Here's how the part is built. I have some questions about the finished solid (model axes, mm). A direction names the side the tool comes from. Coordinates: 2 decimals unless noted, no trailing zeros. Use a Markdown table: item, result. Add a question column.
Item 1: If we mould it in two halves opening along Z, with no side actions, what happens to faces 3 (the flat face through (91.03, -157.32, -249.72)), 4 (the cylindrical face through (-12.77, -1.27, 0.28)), 5 (the flat face through (91.03, -157.32, 249.72))? For each: pulls with the +Z half, pulls with the -Z half, needs draft (parallel to the pull), parting line crosses it, or undercut.
Item 2: If I drill on line 1 along Y through (x, z) = (41, 180); line 2 along Y through (x, z) = (28, -139); line 3 along X through (y, z) = (-101.5, -154), over which ranges is the centre line in solid material (lowest first)? Write a range as from..to.
Item 3: Will these pins go through, and if not, where does the flat tip stop? pin 1 Ø11 at (x, z) = (8.5, 7) entering from +Y; pin 2 Ø4 at (x, z) = (-30.5, 4.5) entering from -Y; pin 3 Ø12.5 at (x, y) = (-18.5, 5) entering from +Z.
Item 4: On a 3-axis mill with a long thin cutter (end or side, diameter ignored), from which of +Z, -Z, +X, -X, +Y, -Y can I reach the whole of each face in a straight line? I mean faces 1 (the flat face through (-12, 2, -20.32)), 2 (the cylindrical face through (-6.17, 25.95, -0.37)). Say none if no direction works.
```python
from build123d import *

# Parameters (mm, degrees)
BOSS_EXTRUDE1_DEPTH = 10.16
SKETCH2_OUTSIDE_W   = 88.516
SKETCH2_OUTSIDE_H   = 38.986
CUT_EXTRUDE1_DEPTH  = 41.64
SKETCH3_R           = 12.7


with BuildPart() as part:
    # Sketch1 → Boss-Extrude1 (new body, symmetric)
    with BuildSketch(Plane(origin=(0, 0, 0), x_dir=(1, 0, 0), z_dir=(0, 1, 0))):
        with BuildLine():
            Line((4.607085175, 20.32), (-28.448, 20.32))
            ThreePointArc((-28.448, 20.32), (-32.938128061, 18.460128061), (-34.798, 13.97))
            Line((-34.798, 13.97), (-34.798, -13.97))
            ThreePointArc((-34.798, -13.97), (-32.938128061, -18.460128061), (-28.448, -20.32))
            Line((-28.448, -20.32), (4.607085175, -20.32))
            ThreePointArc((4.607085175, -20.32), (10.031876423, -19.733940435), (15.206332963, -18.002806293))
            Line((15.206332963, -18.002806293), (30.611774336, -10.928879131))
            ThreePointArc((30.611774336, -10.928879131), (33.846603668, -8.117096905), (35.052, -4.004037244))
            Line((35.052, -4.004037244), (35.052, 4.004037244))
            ThreePointArc((35.052, 4.004037244), (33.846603668, 8.117096905), (30.611774336, 10.928879131))
            Line((30.611774336, 10.928879131), (15.206332963, 18.002806293))
            ThreePointArc((15.206332963, 18.002806293), (10.031876423, 19.733940435), (4.607085175, 20.32))
        make_face()
    extrude(amount=BOSS_EXTRUDE1_DEPTH, both=True)

    # Sketch2 outside → Cut-Extrude1 (cut, through all)
    with BuildSketch(Plane.XY.offset(20.32)):
        with Locations((0.127, 0)):
            Rectangle(SKETCH2_OUTSIDE_W, SKETCH2_OUTSIDE_H)
        with BuildLine():
            Line((-34.798, 10.16), (-24.638, 10.16))
            ThreePointArc((-24.638, 10.16), (-12.998257735, 2.54), (-1.35851547, 10.16))
            Line((-1.35851547, 10.16), (35.052, 10.16))
            Line((35.052, 10.16), (35.052, 6.35))
            Line((35.052, 6.35), (0.913895226, 6.35))
            ThreePointArc((0.913895226, 6.35), (-12.998257735, -1.27), (-26.910410695, 6.35))
            Line((-26.910410695, 6.35), (-34.798, 6.35))
            Line((-34.798, 6.35), (-34.798, 10.16))
        make_face(mode=Mode.SUBTRACT)
    extrude(amount=-CUT_EXTRUDE1_DEPTH, mode=Mode.SUBTRACT)

    # Sweep1: sweep along a curve in space
    with BuildLine() as sweep1_path:
        Line((-12.998257735, 15.24, 0), (-12.998257735, 15.24, 26.090581637))
        ThreePointArc((-12.998257735, 15.24, 26.090581637), (-10.369052155, 5.523370683, 62.566204639), (-3.225691511, -20.876005608, 88.716577691))
        Line((-3.225691511, -20.876005608, 88.716577691), (11.214051911, -74.240274777, 118.469971898))
        ThreePointArc((26.634638374, -101.71962206, 145.570889864), (17.598298945, -90.292217187, 130.430402583), (11.214051911, -74.240274777, 118.469971898))
        Line((26.634638374, -101.71962206, 145.570889864), (91.141742265, -157.48, 249.564780828))
    # Sketch3 → Sweep1 (sweep)
    with BuildSketch(Plane.XY):
        with Locations((-12.998257735, 15.24)):
            Circle(SKETCH3_R)
    sweep(path=sweep1_path.line)

    # Mirror1: part across plane


with BuildPart() as part_1:
    add(part.part)
    add(part.part.mirror(Plane.XY))


solid = part_1.part
```
Ans:
| question | item | result |
|---|---|---|
| 1 | face 3 | pulls with the -Z half |
| 1 | face 4 | undercut |
| 1 | face 5 | pulls with the +Z half |
| 2 | line 1 | y = -130.84..-106.17 |
| 2 | line 2 | y = -112.5..-85.27 |
| 2 | line 3 | x = 16.97..44.31 |
| 3 | pin 1 | stops at y = 10.16 |
| 3 | pin 2 | stops at y = 6.35 |
| 3 | pin 3 | stops at z = 85.97 |
| 4 | face 1 | -Y |
| 4 | face 2 | none |
